```python
from build123d import *

# Parameters (mm, degrees)
BOSS_EXTRUDE1_DEPTH = 2


with BuildPart() as part:
    # Model → Boss-Extrude1 (new body)
    with BuildSketch(Plane.XY):
        Polygon((-240, 125), (240, 125), (238, -125), (-240, -125), align=None)
        with BuildLine():
            Line((-45, 75), (105, 75))
            ThreePointArc((105, 75), (180, 0), (105, -75))
            Line((105, -75), (-45, -75))
            ThreePointArc((-45, -75), (-120, 0), (-45, 75))
        make_face(mode=Mode.SUBTRACT)
    extrude(amount=BOSS_EXTRUDE1_DEPTH)


solid = part.part
```
Check sheet for the modelled part. Datum: model origin and axes. Units: mm. A direction names the side the tool comes from. Give positions to 0.01 mm unless a question says otherwise; leave off trailing zeros. Write each loop counter-clockwise with the first axis right and the second up, starting at its lowest first coordinate (ties: lowest second). Pieces come first, ordered by that corner, then holes. Notation, with made-up numbers: (-34.5, 26) - (-30.5, 26) arc R27 cw to (-30.5, 57) - close; hole circle Ø7 at (-26, 26.25). An arc over 180 degrees is marked (long way). Answer as a JSON object with one key per item and string values. Group by question number.
1) Thickness scan on probe 1 along Y at (x, z) = (30, 1.65); probe 2 along X at (y, z) = (-14.5, 1.8); probe 3 along X at (y, z) = (-39, 1). Record the ranges inside material, lowest first. Write a range as from..to.
2) Sectioned sample at B-B (z = 0.75). Record the cut outline in (x, y).
3) Sectioned sample at C-C (x = -115). Record the cut outline in (y, z).
4) Release check for a two-part mould opening along X. For faces 1 (the face through (3, 85, 0)), 2 (the face through (179.98, 1.65, 0.99)) record: pulls with the +X half, pulls with the -X half, needs draft (parallel to the pull), parting line crosses it, or undercut.
5) Access from +Z, -Z, +X, -X, +Y, -Y to the whole of each face (thin tool, end or side, straight path). Record for faces 3 (the face through (-119.98, -1.65, 0.99)), 4 (the face through (3, 85, 2)).
6) Sectioned sample at A-A (y = 0). Record the cut outline in (x, z), then the cut area to 3 significant figures.
Geometry results:
{
 "1": {"probe 1": "y = -125..-75, 75..125", "probe 2": "x = -240..-118.58, 178.58..238.88", "probe 3": "x = -240..-109.06, 169.06..238.69"},
 "2": {"outline": "(-240, -125) - (238, -125) - (240, 125) - (-240, 125) - close; hole (-45, -75) - (105, -75) arc R75 ccw to (105, 75) - (-45, 75) arc R75 ccw to start"},
 "3": {"outline": "(-125, 0) - (-26.93, 0) - (-26.93, 2) - (-125, 2) - close; (26.93, 0) - (125, 0) - (125, 2) - (26.93, 2) - close"},
 "4": {"face 1": "needs draft", "face 2": "undercut"},
 "5": {"face 3": "+Z, -Z", "face 4": "+Z, +X, -X, +Y, -Y"},
 "6": {"outline": "(-240, 0) - (-120, 0) - (-120, 2) - (-240, 2) - close; (180, 0) - (239, 0) - (239, 2) - (180, 2) - close", "area": "358 mm^2"}
}
